Geometry check sheet. Reference: the model listing, model coordinates, mm. A direction names the side the tool comes from. Give positions to 0.01 mm unless a question says otherwise; leave off trailing zeros. Loops run counter-clockwise (first coordinate to the right, second up) from the corner with the lowest first, then second, coordinate; pieces in that order, holes last.
1. Tool access check on faces 1 (the flat face through (32.5, 0, -5)), 2 (the flat face through (0, -6, -12)), 3 (the flat face through (1.36, -19.89, -10.77)), 4 (the flat face through (7, 0, -10.5)), 5 (the flat face through (-12.6, 0, 0)). Record the directions out of +Z, -Z, +X, -X, +Y, -Y that give a thin tool (end or side, any length) a straight path to the whole face; none if there is none.
2. Cross-section at A-A, the plane y = 0. State how many separate pieces and enclosed holes the cut face has, plus the area to 3 significant figures.
3. Material ranges on L1, parallel to Y at x = 0, z = -7.4; L2, parallel to Y at x = 7.4, z = -7.65; L3, parallel to X at y = -20.5, z = -3.5, recorded low to high.
4. Release check for a two-part mould opening along Y. For faces 6 (the flat face through (-31.1, -0.39, 3.95)), 7 (the flat face through (0, -27.5, -7)), 8 (the cylindrical face through (13.98, -18.11, -3.36)) record: +Y half, -Y half, draft (parallel to the pull), parting line (faces both ways), or undercut.
5. Cross-section at D-D, the plane y = -7. Record the cut outline in (x, z), plus the area to 3 significant figures.
6. Go/stop test with flat-tipped pins: pin 1 Ø2.5 at (x, y) = (-12.5, 17.5) entering from -Z; pin 2 Ø12.5 at (x, y) = (5.5, 4.5) entering from +Z. Record where each tip stops, or that it passes through.
7. Cross-section at B-B, the plane x = -7.4. Record the cut outline in (y, z), plus the area to 3 significant figures.
from build123d import *

# Parameters (mm, degrees)
PAD_DEPTH            = 27.5
SKETCH001_R          = 1.6
POCKET_DEPTH         = 12.001
POCKET_DEPTH_BACK    = -6.001
SKETCH002_R          = 5.1
POCKET001_DEPTH      = 10.5
SKETCH004_W          = 11
SKETCH004_H          = 11
POCKET003_DEPTH      = 27.501
POCKET003_DEPTH_BACK = -27.501
POCKET004_DEPTH      = 2.5


with BuildPart() as part:
    # Sketch → Pad (new body, symmetric)
    with BuildSketch(Plane.XZ):
        with BuildLine():
            Line((-29.664762, 6), (-27.164762, 6))
            ThreePointArc((-27.164762, 6), (-22.5, -7.6), (-17.835238, 6))
            Line((-17.835238, 6), (-12.6, 6))
            Line((-12.6, -6), (-12.6, 6))
            Line((12.6, -6), (-12.6, -6))
            Line((12.6, 6), (12.6, -6))
            Line((12.6, 6), (17.835238, 6))
            ThreePointArc((17.835238, 6), (22.5, -7.6), (27.164762, 6))
            Line((27.164762, 6), (29.664762, 6))
            Line((29.664762, 6), (32.5, 1.95086))
            Line((32.5, 1.95086), (32.5, -12))
            Line((32.5, -12), (-32.5, -12))
            Line((-32.5, -12), (-32.5, 1.95086))
            Line((-32.5, 1.95086), (-29.664762, 6))
        make_face()
    extrude(amount=PAD_DEPTH, both=True)

    # Sketch001 → Pocket (cut, two sides)
    with BuildSketch(Plane.XY) as pocket_sk:
        with Locations((-12.5, 17.5)):
            Circle(SKETCH001_R)
        with Locations((-12.5, -17.5)):
            Circle(SKETCH001_R)
        with Locations((12.5, 17.5)):
            Circle(SKETCH001_R)
        with Locations((12.5, -17.5)):
            Circle(SKETCH001_R)
        with Locations((0, 17.5)):
            Circle(SKETCH001_R)
        with Locations((0, -17.5)):
            Circle(SKETCH001_R)
        Circle(SKETCH001_R)
    extrude(amount=-POCKET_DEPTH, mode=Mode.SUBTRACT)
    extrude(pocket_sk.sketch, amount=-POCKET_DEPTH_BACK, mode=Mode.SUBTRACT)

    # Sketch002 → Pocket001 (cut)
    with BuildSketch(Plane.XY):
        with Locations((-7.4, 0)):
            Circle(SKETCH002_R)
        with Locations((7.4, 0)):
            Circle(SKETCH002_R)
    extrude(amount=-POCKET001_DEPTH, mode=Mode.SUBTRACT)

    # Sketch004 → Pocket003 (cut, two sides)
    with BuildSketch(Plane.XZ) as pocket003_sk:
        with Locations((-22.677406, 5.5)):
            Rectangle(SKETCH004_W, SKETCH004_H)
        with Locations((22.677406, 5.5)):
            Rectangle(SKETCH004_W, SKETCH004_H)
    extrude(amount=-POCKET003_DEPTH, mode=Mode.SUBTRACT)
    extrude(pocket003_sk.sketch, amount=-POCKET003_DEPTH_BACK, mode=Mode.SUBTRACT)

    # Sketch005 (on DatumPlane) → Pocket004 (cut)
    with BuildSketch(Plane.XY.offset(-12)):
        Polygon((-9.75, 15.912287), (-9.75, 19.087713), (-12.5, 20.675426), (-15.25, 19.087713), (-15.25, 15.912287), (-12.5, 14.324574), align=None)
        Polygon((2.75, 15.912287), (2.75, 19.087713), (0, 20.675426), (-2.75, 19.087713), (-2.75, 15.912287), (0, 14.324574), align=None)
        Polygon((15.25, 15.912287), (15.25, 19.087713), (12.5, 20.675426), (9.75, 19.087713), (9.75, 15.912287), (12.5, 14.324574), align=None)
        Polygon((2.75, -1.587713), (2.75, 1.587713), (0, 3.175426), (-2.75, 1.587713), (-2.75, -1.587713), (0, -3.175426), align=None)
        Polygon((-9.75, -15.912287), (-12.5, -14.324574), (-15.25, -15.912287), (-15.25, -19.087713), (-12.5, -20.675426), (-9.75, -19.087713), align=None)
        Polygon((2.75, -19.087713), (2.75, -15.912287), (0, -14.324574), (-2.75, -15.912287), (-2.75, -19.087713), (0, -20.675426), align=None)
        Polygon((15.25, -19.087713), (15.25, -15.912287), (12.5, -14.324574), (9.75, -15.912287), (9.75, -19.087713), (12.5, -20.675426), align=None)
    extrude(amount=POCKET004_DEPTH, mode=Mode.SUBTRACT)


solid = part.part
Result:
1. face 1: +Z, -Z, +X, +Y, -Y
1. face 2: -Z, +X, -X, +Y, -Y
1. face 3: -Z
1. face 4: +Z
1. face 5: +Z, +Y, -Y
2. separate pieces: 4
2. enclosed holes: 0
2. area: 396 mm2
3. L1: y = -27.5 to -19.1, -15.9 to -1.6, 1.6 to 15.9, 19.1 to 27.5
3. L2: y = -27.5 to -5.1, 5.1 to 27.5
3. L3: x = -32.5 to -29.25, -15.75 to -12.6, 12.6 to 15.75, 29.25 to 32.5
4. face 6: draft
4. face 7: -Y half
4. face 8: undercut
5. outline: (-32.5, -12) - (32.5, -12) - (32.5, 1.95) - (29.66, 6) - (28.18, 6) - (28.18, 5.05) arc R7.6 cw (long way) to (17.18, 5.42) - (17.18, 6) - (12.6, 6) - (12.6, -6) - (-12.6, -6) - (-12.6, 6) - (-17.18, 6) - (-17.18, 5.42) arc R7.6 cw (long way) to (-28.18, 5.05) - (-28.18, 6) - (-29.66, 6) - (-32.5, 1.95) - close
5. area: 512 mm2
6. pin 1: passes through
6. pin 2: stops at z = -6
7. outline: (-27.5, -12) - (27.5, -12) - (27.5, -6) - (5.1, -6) - (5.1, -10.5) - (-5.1, -10.5) - (-5.1, -6) - (-27.5, -6) - close
7. area: 284 mm2
